Geometry check sheet. Reference: the model listing, model coordinates, mm. Face numbers are marked on the shaded views. Round coordinates to 2 decimals unless told otherwise and drop trailing zeros. Write each loop counter-clockwise with the first axis right and the second up, starting at its lowest first coordinate (ties: lowest second). Pieces come first, ordered by that corner, then holes. Notation, with made-up numbers: M 8.25,61.5 L 36.25,61.5 A27 cw 36.25,78.5 Z; hole C 37,-11 d4. An arc over 180 degrees is marked long. Put each result on its own line as item: value. Start each with the question number.
(1) Material ranges on probe 1 along Z at (x, y) = (0, 14.5); probe 2 along Z at (x, y) = (0.75, -2); probe 3 along X at (y, z) = (5.5, 12.75), recorded low to high.
(2) Section check D-D on y = 18.75. Record the cut outline in (x, z).
(3) Section check A-A on z = 3. Record the cut outline in (x, y), then the cut area to 4 significant figures.
(4) Section check C-C on y = -3.5. Record the cut outline in (x, z).
(5) Mould release check, pull along X, two halves, no side actions. Record for the marked faces 1, 2, 3 and 4: pulls with the +X half, pulls with the -X half, needs draft (parallel to the pull), parting line crosses it, or undercut.
(6) Section check B-B on y = 6.5. Record the cut outline in (x, z), then the cut area to 3 significant figures.
(7) Gauge pin test, flat ends, axial feed: pin 1 (4 mm diameter, centred on x = 5.5, y = 13.5, fed in from +Z); pin 2 (4.5 mm diameter, centred on y = -2, z = 7.5, fed in from -X); pin 3 (2.5 mm diameter, centred on x = 0, z = 7.5, fed in from -Y). Record the tip position at first contact, or that the pin passes through.
from build123d import *
from build123d.topology import SkipClean

# Parameters (mm, degrees)
SKETCH1_W           = 6.5
SKETCH1_H           = 14
BOSS_EXTRUDE1_DEPTH = 15
FILLET1_R           = 10
SKETCH2_R           = 2
CUT_EXTRUDE1_DEPTH  = 18.783419244
SKETCH4_R           = 7.5
BOSS_EXTRUDE2_DEPTH = 15
SKETCH6_W           = 7
SKETCH6_H           = 12.68
CUT_EXTRUDE2_DEPTH  = 28.663152387
CUT_EXTRUDE3_DEPTH  = 23.5
SKETCH11_R          = 1.25
CUT_EXTRUDE7_DEPTH  = 24
BOSS_EXTRUDE3_START = 12.68
SKETCH12_R          = 1.25
BOSS_EXTRUDE3_DEPTH = 12.68
SKETCH13_R          = 1.5
CUT_EXTRUDE8_DEPTH  = 6


with BuildPart() as part:
    # Sketch1 → Boss-Extrude1 (new body)
    with BuildSketch(Plane.XY):
        Rectangle(SKETCH1_W, SKETCH1_H)
    extrude(amount=BOSS_EXTRUDE1_DEPTH)

    # Fillet1
    fillet1_edges = [part.edges().sort_by_distance(p)[0] for p in [
        (0, -7, 15),
    ]]
    fillet(fillet1_edges, radius=FILLET1_R)

    # Sketch2 → Cut-Extrude1 (cut, through all)
    with BuildSketch(Plane(origin=(3.25, 0, 0), x_dir=(0, 0, -1), z_dir=(1, 0, 0))):
        with Locations(Location((-7.5, -2, 0), (0, 0, 90))):
            Circle(SKETCH2_R)
    extrude(amount=-CUT_EXTRUDE1_DEPTH, mode=Mode.SUBTRACT)

    # Sketch4 → Boss-Extrude2 (add)
    with BuildSketch(Plane(origin=(0, 7, 0), x_dir=(1, 0, 0), z_dir=(0, 1, 0))):
        with Locations(Location((0, -7.5, 0), (0, 0, 270))):
            Circle(SKETCH4_R)
    extrude(amount=BOSS_EXTRUDE2_DEPTH)

    # Sketch6 → Cut-Extrude2 (cut, through all)
    with BuildSketch(Plane(origin=(0, 0, 0), x_dir=(-1, 0, 0), z_dir=(0, 0, -1))):
        with Locations((0, 15.66)):
            Rectangle(SKETCH6_W, SKETCH6_H)
    extrude(amount=-CUT_EXTRUDE2_DEPTH, mode=Mode.SUBTRACT)

    # Sketch7 → Cut-Extrude3 (cut, through all)
    with BuildSketch(Plane(origin=(0, 7, 0), x_dir=(1, 0, 0), z_dir=(0, 1, 0))):
        with BuildLine():
            ThreePointArc((0, -15), (-1.666673801, -14.812468697), (-3.25, -14.259252917))
            Line((-3.25, -14.259252917), (-3.25, -15))
            Line((-3.25, -15), (0, -15))
        make_face()
        with BuildLine():
            ThreePointArc((3.25, -14.259252917), (1.666673801, -14.812468697), (0, -15))
            Line((0, -15), (3.25, -15))
            Line((3.25, -15), (3.25, -14.259252917))
        make_face()
        with BuildLine():
            ThreePointArc((-3.25, -0.740747083), (-1.666673801, -0.187531303), (0, 0))
            Line((0, 0), (-3.25, 0))
            Line((-3.25, 0), (-3.25, -0.740747083))
        make_face()
        with BuildLine():
            Line((3.25, 0), (0, 0))
            ThreePointArc((0, 0), (1.666673801, -0.187531303), (3.25, -0.740747083))
            Line((3.25, -0.740747083), (3.25, 0))
        make_face()
    extrude(amount=-CUT_EXTRUDE3_DEPTH, mode=Mode.SUBTRACT)

    # Sketch11 → Cut-Extrude7 (cut)
    with BuildSketch(Plane.XZ.offset(7)):
        with Locations(Location((0, 12.74882624, 0), (0, 0, 270))):
            Circle(SKETCH11_R)
        with Locations(Location((0, 3, 0), (0, 0, 270))):
            Circle(SKETCH11_R)
    extrude(amount=-CUT_EXTRUDE7_DEPTH, mode=Mode.SUBTRACT)

    # Sketch12 → Boss-Extrude3 (add)
    with SkipClean():  # the faces are left unmerged after this step: merging them gives an invalid solid
        with BuildSketch(Plane(origin=(0, 9.32, 0), x_dir=(1, 0, 0), z_dir=(0, 1, 0)).offset(BOSS_EXTRUDE3_START)):
            with BuildLine():
                Line((3.5, -14.133249581), (3.5, -0.866750419))
                ThreePointArc((3.5, -0.866750419), (0, 0), (-3.5, -0.866750419))
                Line((-3.5, -0.866750419), (-3.5, -14.133249581))
                ThreePointArc((-3.5, -14.133249581), (0, -15), (3.5, -14.133249581))
            make_face()
            with Locations(Location((0, -3, 0), (0, 0, 90))):
                Circle(SKETCH12_R, mode=Mode.SUBTRACT)
            with Locations(Location((0, -12.74882624, 0), (0, 0, 90))):
                Circle(SKETCH12_R, mode=Mode.SUBTRACT)
        extrude(amount=-BOSS_EXTRUDE3_DEPTH)

    # Sketch13 → Cut-Extrude8 (cut)
    with SkipClean():  # the faces are left unmerged after this step: merging them gives an invalid solid
        with BuildSketch(Plane(origin=(0, 22, 0), x_dir=(1, 0, 0), z_dir=(0, 1, 0))):
            with Locations(Location((0, -7.5, 0), (0, 0, 270))):
                Circle(SKETCH13_R)
        extrude(amount=-CUT_EXTRUDE8_DEPTH, mode=Mode.SUBTRACT)


solid = part.part
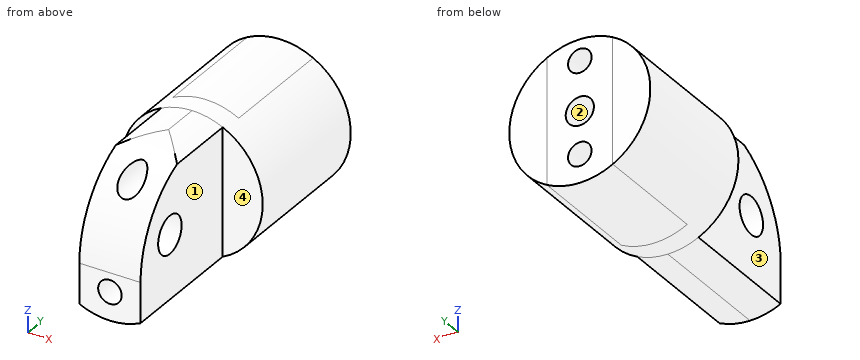
Answers follow:
1. probe 1: z = 0 to 1.75, 4.25 to 11.5, 14 to 15
1. probe 2: z = 0.04 to 2, 4 to 5.5, 9.5 to 11.75
1. probe 3: x = -3.25 to -1.25, 1.25 to 3.25
2. outline: C 0,7.5 d15; hole C 0,7.5 d3; hole C 0,3 d2.5; hole C 0,12.75 d2.5
3. outline: M -6,7 L -3.25,7 L -3.25,-7 L -1.25,-7 L -1.25,22 L -6,22 Z; M 1.25,-7 L 3.25,-7 L 3.25,7 L 6,7 L 6,22 L 1.25,22 Z
3. area: 198.5 mm^2
4. outline: M -3.25,0.74 A7.5 ccw 3.25,0.74 L 3.25,6.18 L -3.25,6.18 Z; M -3.25,8.82 L 3.25,8.82 L 3.25,12.6 L 1.24,12.6 A1.25 cw -1.24,12.6 L -3.25,12.6 Z; hole C 0,3 d2.5
5. face 1: pulls with the +X half
5. face 2: undercut
5. face 3: pulls with the -X half
5. face 4: needs draft
6. outline: M -3.25,0.74 A7.5 ccw 3.25,0.74 L 3.25,14.26 A7.5 ccw -3.25,14.26 Z; hole C 0,3 d2.5; hole C 0,12.75 d2.5
6. area: 84.5 mm^2
7. pin 1: stops at z = 14.13
7. pin 2: stops at x = -3.25
7. pin 3: stops at y = -6.92
